Input: part model. Units: mm. Frame: model coordinates. A direction names the side the tool comes from. Round coordinates to 2 decimals unless told otherwise and drop trailing zeros. Loops run counter-clockwise (first coordinate to the right, second up) from the corner with the lowest first, then second, coordinate; pieces in that order, holes last. Notation, with made-up numbers: (54, 45.5) -> (71, 45.5) arc R32 ccw to (71, 84.5) -> close; hole circle Ø9 at (47.25, -4). An arc over 180 degrees is marked (long way). Answer as a JSON object with one key per item and string values. Group by question number.
Item 1: Section query A-A on y = -0.5. Return loops of the section in (x, z), and give its area (3 significant figures).
Item 2: Material intervals for line 1 (Y direction, x = -2, z = 0.7); line 2 (X direction, y = 2, z = 1.6); line 3 (Y direction, x = 1, z = 2.75), sorted ascending. Write a range as [from, to].
Item 3: Pin query (flat end, axial travel): pin 1 (0.6 mm diameter, centred on x = 2, z = 2, fed in from +Y); pin 2 (0.5 mm diameter, centred on x = 2, z = 2.5, fed in from -Y). Return the tip coordinate at first contact, or that it passes through.
Item 4: Draft query along X for faces 1 (the flat face through (5, 55, 2)), 2 (the flat face through (2, 44.7, 2)), 3 (the flat face through (-2, 44.7, 2)), 4 (the flat face through (7.5, 25, 2)). Return one class per face: released by +X, released by -X, zero draft, split by the parting line, or undercut.
Item 5: Set-up query: faces 5 (the flat face through (-1.5, 48, 2)), 6 (the flat face through (2, 47, 2)), 7 (the flat face through (-1.5, 8, 2)). Return all of +Z, -Z, +X, -X, +Y, -Y with unobstructed straight access to the full face (end or side cutting, diameter ignored); none if empty.
from build123d import *

# Parameters (mm, degrees)
BOSS_EXTRU_1_DEPTH = 5


with BuildPart() as part:
    # Esquisse1 → Boss.-Extru.1 (new body)
    with BuildSketch(Plane.XY):
        Polygon((-7.5, 50), (-7.5, 25), (7.5, 25), (7.5, 50), (7.5, 55), (2.5, 55), (2.5, 50), (1.5, 50), (1.5, 47), (2.6, 47), (2.6, 44.7), (1.5, 44.7), (1.5, 40), (-1.5, 40), (-1.5, 44.7), (-2.6, 44.7), (-2.6, 47), (-1.5, 47), (-1.5, 50), (-2.5, 50), (-2.5, 55), (-7.5, 55), align=None)
        Polygon((-7.5, 25), (-7.5, 0), (-7.5, -5), (-2.5, -5), (-2.5, 0), (-1.5, 0), (-1.5, 3), (-2.6, 3), (-2.6, 5.3), (-1.5, 5.3), (-1.5, 10), (1.5, 10), (1.5, 5.3), (2.6, 5.3), (2.6, 3), (1.5, 3), (1.5, 0), (2.5, 0), (2.5, -5), (7.5, -5), (7.5, 0), (7.5, 25), align=None)
    extrude(amount=BOSS_EXTRU_1_DEPTH)


solid = part.part
Solved:
{
 "1": {"outline": "(-7.5, 0) -> (-2.5, 0) -> (-2.5, 5) -> (-7.5, 5) -> close; (2.5, 0) -> (7.5, 0) -> (7.5, 5) -> (2.5, 5) -> close", "area": "50.0 mm²"},
 "2": {"line 1": "[0, 3], [5.3, 44.7], [47, 50]", "line 2": "[-7.5, -1.5], [1.5, 7.5]", "line 3": "[10, 40]"},
 "3": {"pin 1": "y = 50", "pin 2": "y = 0"},
 "4": {"face 1": "zero draft", "face 2": "undercut", "face 3": "undercut", "face 4": "released by +X"},
 "5": {"face 5": "+Z, -Z, +Y", "face 6": "+Z, -Z", "face 7": "+Z, -Z, -Y"}
}
